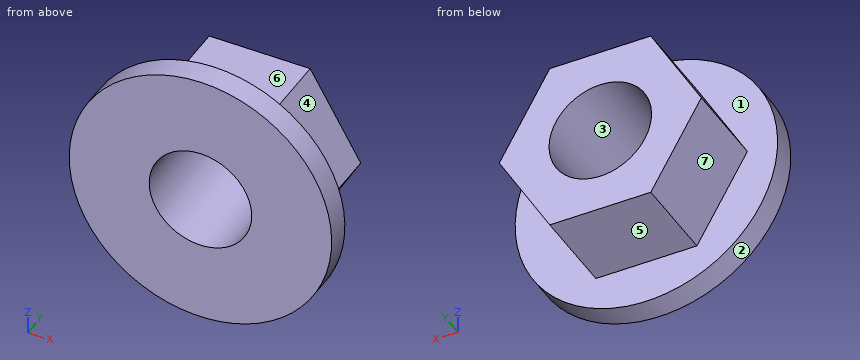
```python
from build123d import *

# Parameters (mm, degrees)
HEX_NUT_DEPTH                     = 3.5
NUT_FLANGE_SKETCH_R               = 5.25
NUT_FLANGE_DEPTH                  = 1
M4_INTERNAL_THREAD_BLANK_SKETCH_R = 2.05
M4_INTERNAL_THREAD_BLANK_DEPTH    = 4.7


with BuildPart() as part:
    # Hex Nut Sketch → Hex Nut (new body)
    with BuildSketch(Plane(origin=(0, 138.5, 0), x_dir=(1, 0, 0), z_dir=(0, 1, 0))):
        Polygon((-16.250199362, 0), (-18.270925304, -3.5), (-22.312377188, -3.5), (-24.33310313, 0), (-22.312377188, 3.5), (-18.270925304, 3.5), align=None)
    extrude(amount=-HEX_NUT_DEPTH)

    # Nut Flange Sketch → Nut Flange (add)
    with BuildSketch(Plane(origin=(0, 135, 0), x_dir=(1, 0, 0), z_dir=(0, 1, 0))):
        with Locations(Location((-20.291651246, 0, 0), (0, 0, 270))):
            Circle(NUT_FLANGE_SKETCH_R)
    extrude(amount=-NUT_FLANGE_DEPTH)

    # M4 Internal Thread Blank Sketch → M4 Internal Thread Blank (cut)
    with BuildSketch(Plane(origin=(0, 138.6, 0), x_dir=(1, 0, 0), z_dir=(0, 1, 0))):
        with Locations(Location((-20.291651246, 0, 0), (0, 0, 270))):
            Circle(M4_INTERNAL_THREAD_BLANK_SKETCH_R)
    extrude(amount=-M4_INTERNAL_THREAD_BLANK_DEPTH, mode=Mode.SUBTRACT)


solid = part.part
```
Verification items for the finished model (mm, model axes). Face numbers are marked on the shaded views. A direction names the side the tool comes from. Give positions to 0.01 mm unless a question says otherwise; leave off trailing zeros. Order: outer loops, then holes, each group sorted by start corner. A loop starts at its lowest first (then second) coordinate and runs counter-clockwise, first axis right, second up. Notation, with made-up numbers: (-0.5, 71) -> (24.5, 71) arc R10 ccw to (24.5, 87) -> close; hole circle Ø6 at (3.5, 74). An arc over 180 degrees is marked (long way). Use a Markdown table: item, result.
1) Depth check by flat-ended pin: pin 1 Ø1.8 at (x, y) = (-19.5, 137) entering from -Z; pin 2 Ø2 at (x, y) = (-19, 135.5) entering from -Z; pin 3 Ø4.5 at (x, z) = (-20.29, 0) entering from +Y; pin 4 Ø2 at (y, z) = (135, 2.5) entering from +X. Enter the tip coordinate at first touch or a pass-through.
Results:
| item | result |
|---|---|
| pin 1 | z = -3.5 |
| pin 2 | z = -5.23 |
| pin 3 | y = 138.5 |
| pin 4 | x = -15.26 |
2) Mould release check, pull along Z, two halves, no side actions. Record for the marked faces 1, 2, 3 and 4: pulls with the +Z half, pulls with the -Z half, needs draft (parallel to the pull), parting line crosses it, or undercut.
Results:
| item | result |
|---|---|
| face 1 | needs draft |
| face 2 | parting line crosses it |
| face 3 | undercut |
| face 4 | pulls with the +Z half |
3) Section check D-D, the plane z = -3.25. Record the boundary of the cut face in (x, y), then the cut area to 3 significant figures.
Results:
| item | result |
|---|---|
| outline | (-24.41, 134) -> (-16.17, 134) -> (-16.17, 135) -> (-18.13, 135) -> (-18.13, 138.5) -> (-22.46, 138.5) -> (-22.46, 135) -> (-24.41, 135) -> close |
| area | 23.4 mm² |
4) Material ranges on probe 1 along Z at (x, y) = (-21.5, 136.8); probe 2 along Y at (x, z) = (-20.5, -4.5); probe 3 along X at (y, z) = (136.65, 1.75), recorded low to high.
Results:
| item | result |
|---|---|
| probe 1 | -3.5 to -1.66, 1.66 to 3.5 |
| probe 2 | 134 to 135 |
| probe 3 | -23.32 to -21.36, -19.22 to -17.26 |
5) Section check A-A, the plane x = -18.75. Record the boundary of the cut face in (y, z), then the cut area to 3 significant figures.
Results:
| item | result |
|---|---|
| outline | (134, -5.02) -> (135, -5.02) -> (135, -3.5) -> (138.5, -3.5) -> (138.5, -1.35) -> (134, -1.35) -> close; (134, 1.35) -> (138.5, 1.35) -> (138.5, 3.5) -> (135, 3.5) -> (135, 5.02) -> (134, 5.02) -> close |
| area | 22.4 mm² |
6) Section check B-B, the plane y = 137.3. Record the boundary of the cut face in (x, z).
Results:
| item | result |
|---|---|
| outline | (-24.33, 0) -> (-22.31, -3.5) -> (-18.27, -3.5) -> (-16.25, 0) -> (-18.27, 3.5) -> (-22.31, 3.5) -> close; hole circle Ø4.1 at (-20.29, 0) |
7) Section check C-C, the plane x = -23.75. Record the boundary of the cut face in (y, z), then the cut area to 3 significant figures.
Results:
| item | result |
|---|---|
| outline | (134, -3.95) -> (135, -3.95) -> (135, -1.01) -> (138.5, -1.01) -> (138.5, 1.01) -> (135, 1.01) -> (135, 3.95) -> (134, 3.95) -> close |
| area | 15.0 mm² |
8) Tool access check on the marked faces 5, 6 and 7. Record the directions out of +Z, -Z, +X, -X, +Y, -Y that give a thin tool (end or side, any length) a straight path to the whole face; none if there is none.
Results:
| item | result |
|---|---|
| face 5 | -Z, +X, -X, +Y |
| face 6 | +Z, +X, -X, +Y |
| face 7 | -Z, -X, +Y |
